from build123d import *

# Parameters (mm, degrees)
F0_R     = 8.255
F1_DEPTH = 25.4
F2_R     = 5.08
F3_DEPTH = 6.35
F5_DEPTH = 3.048
F6_R     = 1.905


with BuildPart() as f1:
    # F0 (on Top) → F1 (new body)
    with BuildSketch(Plane.XY):
        Circle(F0_R)
    extrude(amount=F1_DEPTH)

    # F2 (on face) → F3 (join)
    with BuildSketch(Plane.XY.offset(25.4)):
        Circle(F2_R)
    extrude(amount=F3_DEPTH)

    # F4 (on face) → F5 (cut)
    with BuildSketch(Plane.XY.offset(31.75)):
        Polygon((1.283161, 2.2225), (-1.283161, 2.2225), (-2.566322, 0), (-1.283161, -2.2225), (1.283161, -2.2225), (2.566322, 0), align=None)
    extrude(amount=-F5_DEPTH, mode=Mode.SUBTRACT)

    # F6
    f6_edges = [f1.edges().sort_by_distance(p)[0] for p in [
        (-8.255, 0, 25.4),
        (-5.08, 0, 31.75),
    ]]
    fillet(f6_edges, radius=F6_R)


solid = f1.part
Could you check a few things on this model? Use its own coordinates, in mm. A direction names the side the tool comes from. Round coordinates to 2 decimals unless told otherwise and drop trailing zeros. Loops run counter-clockwise (first coordinate to the right, second up) from the corner with the lowest first, then second, coordinate; pieces in that order, holes last. Notation, with made-up numbers: (72, 26) - (92, 26) arc R16 ccw to (92, 40) - close; hole circle Ø2 at (25, 10). An arc over 180 degrees is marked (long way). Write item = value, one per line.
1) On a 3-axis mill with a long thin cutter (end or side, diameter ignored), from which of +Z, -Z, +X, -X, +Y, -Y can I reach the whole of each face in a straight line? I mean faces 1 (the cylindrical face through (-0.661, 5.037, 27.591)), 2 (the flat face through (2, -2, 31.75)). Say none if no direction works.
Computed:
face_1 = +Z
face_2 = +Z, +X, -X, +Y, -Y
2) I need wall thicknesses on line 1 along Y through (x, z) = (6.5, 3); line 2 along Z through (x, y) = (3, -5.5); line 3 along Z through (x, y) = (-3.25, 0.25). Which ranges of each line are inside material? Lowest first, please. Write a range as from..to.
Computed:
line_1 = -5.09..5.09
line_2 = 0..25.4
line_3 = 0..31.75
3) I'm going to push flat-ended pins straight in: P1, Ø4, axis at y = -5.5, z = 24, coming from the -X side; P2, Ø3, axis at x = -0.5, z = 30.5, coming from the +Y side; P3, Ø4, axis at y = -5, z = 17.5, coming from the +X side. Where does each tip first touch, or does it pass through?
Computed:
P1 = -7.45
P2 = 5.08
P3 = 7.69
4) If we mould it in two halves opening along X, with no side actions, what happens to faces 3 (the cylindrical face through (7.874, 2.48, 11.583)), 4 (the flat face through (2, 5, 25.4)), 5 (the flat face through (-1.916, 1.127, 30.247)), 6 (the flat face through (0, 0, 28.702))? For each: pulls with the +X half, pulls with the -X half, needs draft (parallel to the pull), parting line crosses it, or undercut.
Computed:
face_3 = parting line crosses it
face_4 = needs draft
face_5 = undercut
face_6 = undercut
5) Imagine slicing it at B-B (z = 17). Please give me the cut outline in (x, y) (3 decimals), and give its area (3 significant figures).
Computed:
outline = circle Ø16.51 at (0, 0)
area = 214 mm2
